Work out the finished part from the listing and answer in its coordinate system (mm). A direction names the side the tool comes from. Round coordinates to 2 decimals unless told otherwise and drop trailing zeros. Write each loop counter-clockwise with the first axis right and the second up, starting at its lowest first coordinate (ties: lowest second). Pieces come first, ordered by that corner, then holes. Notation, with made-up numbers: (12, 39) - (24, 39) arc R13 ccw to (24, 58) - close; hole circle Ø7 at (-16.75, 59). An arc over 180 degrees is marked (long way). Answer as a JSON object with one key per item and string values.
```python
from build123d import *

# Parameters (mm, degrees)
EXTRUDE_1_DEPTH     = 9
SKETCH_3_R          = 1.4
CUT_EXTRUDE_1_DEPTH = 29.436068645
FILLET_1_R          = 4
EXTRUDE_START       = 2
EXTRUDE_2_DEPTH     = 2


with BuildPart() as part:
    # 草图1 → 凸台-拉伸1 (new body)
    with BuildSketch(Plane.XY):
        with BuildLine():
            Line((-6.1, -20), (-2.1, -20))
            Line((-2.1, -20), (-2.1, -12))
            Line((-2.1, -12), (2.1, -12))
            Line((2.1, -12), (2.1, -20))
            Line((2.1, -20), (6.1, -20))
            Line((6.1, -20), (6.1, -10.333924714))
            ThreePointArc((6.1, -10.333924714), (10.421132376, -5.949789912), (12, 0))
            Line((12, 0), (10.15, 0))
            ThreePointArc((10.15, 0), (0, -10.15), (-10.15, 0))
            Line((-10.15, 0), (-12, 0))
            ThreePointArc((-12, 0), (-10.421132376, -5.949789912), (-6.1, -10.333924714))
            Line((-6.1, -10.333924714), (-6.1, -20))
        make_face()
    extrude(amount=EXTRUDE_1_DEPTH)

    # 草图3 → 切除-拉伸1 (cut, through all)
    with BuildSketch(Plane.ZY.offset(6.1)):
        with Locations(Location((4.5, -16, 0), (0, 0, 270))):
            Circle(SKETCH_3_R)
    extrude(amount=-CUT_EXTRUDE_1_DEPTH, mode=Mode.SUBTRACT)

    # 圆角1
    fillet_1_edges = [part.edges().sort_by_distance(p)[0] for p in [
        (-6.1, -10.333924714, 4.5),
        (6.1, -10.333924714, 4.5),
    ]]
    fillet(fillet_1_edges, radius=FILLET_1_R)

    # 草图4 → 凸台-拉伸2 (add)
    with BuildSketch(Plane(origin=(0, 0, 0), x_dir=(-1, 0, 0), z_dir=(0, 0, -1)).offset(EXTRUDE_START)):
        with BuildLine():
            ThreePointArc((12, 0), (0, 12), (-12, 0))
            Line((-12, 0), (-10.15, 0))
            ThreePointArc((-10.15, 0), (0, -10.15), (10.15, 0))
            Line((10.15, 0), (12, 0))
        make_face()
        with BuildLine():
            Line((-2.1, -20), (-2.1, -12))
            Line((-2.1, -12), (2.1, -12))
            Line((2.1, -12), (2.1, -20))
            Line((2.1, -20), (6.1, -20))
            Line((6.1, -20), (6.1, -12.409270728))
            ThreePointArc((6.1, -12.409270728), (6.487521626, -10.691714324), (7.575, -9.306953046))
            ThreePointArc((7.575, -9.306953046), (10.837435121, -5.152669211), (12, 0))
            Line((12, 0), (10.15, 0))
            ThreePointArc((10.15, 0), (0, -10.15), (-10.15, 0))
            Line((-10.15, 0), (-12, 0))
            ThreePointArc((-12, 0), (-10.837435121, -5.152669211), (-7.575, -9.306953046))
            ThreePointArc((-7.575, -9.306953046), (-6.487521626, -10.691714324), (-6.1, -12.409270728))
            Line((-6.1, -12.409270728), (-6.1, -20))
            Line((-6.1, -20), (-2.1, -20))
        make_face()
    extrude(amount=-EXTRUDE_2_DEPTH)


solid = part.part
```
Item 1: Determine the mould class of faces 1 (the flat face through (0, -12, 3)), 2 (the cylindrical face through (-4.13, -14.89, 3.65)), 3 (the flat face through (2.1, -17, 3)), 4 (the cylindrical face through (4.07, -14.89, 3.65)) for opening direction Y: pulls with the +Y half, pulls with the -Y half, needs draft (parallel to the pull), parting line crosses it, or undercut.
Results found:
{"face 1": "pulls with the -Y half", "face 2": "undercut", "face 3": "needs draft", "face 4": "undercut"}
Item 2: Consider line 1 along X through (y, z) = (-18, 0.5); line 2 along Z through (x, y) = (3.8, -16); line 3 along Z through (x, y) = (7.75, -1.5). Determine where each line is inside the solid, lowest interval first.
Results found:
{"line 1": "-6.1 to -2.1, 2.1 to 6.1", "line 2": "-2 to 3.1, 5.9 to 9", "line 3": "-2 to 0"}
Item 3: A cutting plane is placed at D-D (z = 2). Write down the section's boundary in (x, y) (3 decimals).
Results found:
{"outline": "(-12, 0) arc R12 ccw to (-7.575, -9.307) arc R4 cw to (-6.1, -12.409) - (-6.1, -20) - (-2.1, -20) - (-2.1, -12) - (2.1, -12) - (2.1, -20) - (6.1, -20) - (6.1, -12.409) arc R4 cw to (7.575, -9.307) arc R12 ccw to (12, 0) - (10.15, 0) arc R10.15 cw to (-10.15, 0) - close"}
Item 4: Each of these flat-tipped pins is pushed along its axis until it touches: P1, Ø1.5, axis at x = -11, z = 5.5, coming from the +Y side; P2, Ø6.5, axis at y = -17.5, z = 2, coming from the +X side; P3, Ø3, axis at x = -3.5, z = 6.5, coming from the +Y side. Where does it stop, or does it pass through?
Results found:
{"P1": "y = 0", "P2": "x = 6.1", "P3": "y = -8.83"}
Item 5: For faces 5 (the flat face through (6.1, -17, 3)), 6 (the flat face through (-2.1, -15, 3)), 7 (the flat face through (11, 0, 4)), 8 (the flat face through (-6.1, -17, 3)), 9 (the flat face through (0, 1, 0)), determine the directions among +Z, -Z, +X, -X, +Y, -Y from which every point of the face is accessible in a straight line to the end or side of a thin tool.
Results found:
{"face 5": "+Z, -Z, +X, -Y", "face 6": "+Z, -Z, -Y", "face 7": "+Z, +X, -X, +Y", "face 8": "+Z, -Z, -X, -Y", "face 9": "+Z, +Y"}
Item 6: A cutting plane is placed at A-A (y = -16). Write down the section's boundary in (x, z), and give its area (3 significant figures).
Results found:
{"outline": "(-6.1, -2) - (-2.1, -2) - (-2.1, 3.1) - (-6.1, 3.1) - close; (-6.1, 5.9) - (-2.1, 5.9) - (-2.1, 9) - (-6.1, 9) - close; (2.1, -2) - (6.1, -2) - (6.1, 3.1) - (2.1, 3.1) - close; (2.1, 5.9) - (6.1, 5.9) - (6.1, 9) - (2.1, 9) - close", "area": "65.6 mm²"}
Item 7: A cutting plane is placed at C-C (x = 4.5). Write down the section's boundary in (y, z), and give its area (3 significant figures).
Results found:
{"outline": "(-20, -2) - (11.12, -2) - (11.12, 0) - (-9.1, 0) - (-9.1, 9) - (-20, 9) - close; hole circle Ø2.8 at (-16, 4.5)", "area": "154 mm²"}
Item 8: A cutting plane is placed at B-B (z = 4.5). Write down the section's boundary in (x, y) (3 decimals).
Results found:
{"outline": "(-12, 0) arc R12 ccw to (-7.575, -9.307) arc R4 cw to (-6.1, -12.409) - (-6.1, -14.6) - (-2.1, -14.6) - (-2.1, -12) - (2.1, -12) - (2.1, -14.6) - (6.1, -14.6) - (6.1, -12.409) arc R4 cw to (7.575, -9.307) arc R12 ccw to (12, 0) - (10.15, 0) arc R10.15 cw to (-10.15, 0) - close; (-6.1, -20) - (-2.1, -20) - (-2.1, -17.4) - (-6.1, -17.4) - close; (2.1, -20) - (6.1, -20) - (6.1, -17.4) - (2.1, -17.4) - close"}
